Part model, mm, in its own coordinate system. A direction names the side the tool comes from. Coordinates: 2 decimals unless noted, no trailing zeros. Loops run counter-clockwise (first coordinate to the right, second up) from the corner with the lowest first, then second, coordinate; pieces in that order, holes last. Notation, with made-up numbers: (-29.75, 81.5) - (25.25, 81.5) arc R26 ccw to (25.25, 111.5) - close; hole circle Ø9 at (81, 89.25). An arc over 180 degrees is marked (long way). Answer as CSV lines item,"result".
from build123d import *

# Parameters (mm, degrees)
BOSS_EXTRUDE1_DEPTH     = 5
BOSS_EXTRUDE1_DRAFT     = 20
MIRROR1_COPY_1_DEPTH    = 5
MIRROR1_COPY_1_DRAFT    = 20
FILLET1_R               = 10
CUT_EXTRUDE1_DEPTH      = 0.5
SKETCH3_R               = 3.628485538
CUT_EXTRUDE2_DEPTH      = 1
CUT_EXTRUDE2_DRAFT      = -20
SKETCH4_W               = 69.290584113
SKETCH4_H               = 7.5
BOSS_EXTRUDE2_DEPTH     = 25
CUT_EXTRUDE3_DEPTH      = 79.012436871
CUT_EXTRUDE3_DEPTH_BACK = 70


with BuildPart() as part:
    # Sketch1 → Boss-Extrude1 (with draft: the straight prism first)
    with BuildSketch(Plane.XY):
        with BuildLine():
            ThreePointArc((-20.793357934, 20), (-40.793357934, 0), (-20.793357934, -20))
            Line((-20.793357934, -20), (9.206642066, -20))
            ThreePointArc((9.206642066, -20), (29.206642066, 0), (9.206642066, 20))
            Line((9.206642066, 20), (-20.793357934, 20))
        make_face()
    extrude(amount=-BOSS_EXTRUDE1_DEPTH)
    # Boss-Extrude1: the draft: its side faces are tilted about the plane it starts from
    boss_extrude1_sides = [part.faces().sort_by_distance(p)[0] for p in [
        (-5.793357934, -20, -2.5),
        (29.206642066, 0, -2.5),
        (-5.793357934, 20, -2.5),
        (-40.793357934, 0, -2.5),
    ]]
    draft(boss_extrude1_sides, Plane.XY, BOSS_EXTRUDE1_DRAFT)


with BuildPart() as mirror1_copy_1_tool:
    # Mirror1 copy 1 sketch → Mirror1 copy 1 (with draft: the straight prism first)
    with BuildSketch(Plane(origin=(0, 0, -10), x_dir=(1, 0, 0), z_dir=(0, 0, -1))):
        with BuildLine():
            ThreePointArc((-20.793357934, -20), (-40.793357934, 0), (-20.793357934, 20))
            Line((-20.793357934, 20), (9.206642066, 20))
            ThreePointArc((9.206642066, 20), (29.206642066, 0), (9.206642066, -20))
            Line((9.206642066, -20), (-20.793357934, -20))
        make_face()
    extrude(amount=-MIRROR1_COPY_1_DEPTH)
    # Mirror1 copy 1: the draft: its side faces are tilted about the plane it starts from
    mirror1_copy_1_sides = [mirror1_copy_1_tool.faces().sort_by_distance(p)[0] for p in [
        (-5.793357934, -20, -7.5),
        (29.206642066, 0, -7.5),
        (-5.793357934, 20, -7.5),
        (-40.793357934, 0, -7.5),
    ]]
    draft(mirror1_copy_1_sides, Plane(origin=(0, 0, -10), x_dir=(1, 0, 0), z_dir=(0, 0, -1)), MIRROR1_COPY_1_DRAFT)


with BuildPart() as part_1:
    add(part.part)

    # Mirror1 copy 1: add mirror1_copy_1_tool
    add(mirror1_copy_1_tool.part)

    # Fillet1
    fillet1_edges = [part_1.edges().sort_by_distance(p)[0] for p in [
        (31.026493238, 0, -5),
        (-5.793357934, 21.819851171, -5),
        (-42.613209105, 0, -5),
        (-5.793357934, -21.819851171, -5),
    ]]
    fillet(fillet1_edges, radius=FILLET1_R)

    # Sketch2 → Cut-Extrude1 (cut)
    with BuildSketch(Plane(origin=(0, 0, -10), x_dir=(-1, 0, 0), z_dir=(0, 0, -1))):
        with BuildLine():
            Line((-17.429161642, 6.728379016), (-2.895862967, 6.728379016))
            ThreePointArc((-2.895862967, 6.728379016), (3.832516049, 0), (-2.895862967, -6.728379016))
            Line((-2.895862967, -6.728379016), (-17.429161642, -6.728379016))
            ThreePointArc((-17.429161642, -6.728379016), (-24.157540659, 0), (-17.429161642, 6.728379016))
        make_face()
    extrude(amount=-CUT_EXTRUDE1_DEPTH, mode=Mode.SUBTRACT)


with BuildPart() as cut_extrude2_tool:
    # Sketch3 → Cut-Extrude2 (with draft: the straight prism first)
    with BuildSketch(Plane(origin=(0, 0, -9.5), x_dir=(-1, 0, 0), z_dir=(0, 0, -1))):
        with Locations((-17.44999147, 0)):
            Circle(SKETCH3_R)
    extrude(amount=-CUT_EXTRUDE2_DEPTH)
    # Cut-Extrude2: the draft: its side faces are tilted about the plane it starts from
    cut_extrude2_sides = [cut_extrude2_tool.faces().sort_by_distance(p)[0] for p in [
        (21.078477008, 0, -9),
    ]]
    draft(cut_extrude2_sides, Plane(origin=(0, 0, -9.5), x_dir=(-1, 0, 0), z_dir=(0, 0, -1)), CUT_EXTRUDE2_DRAFT)


with BuildPart() as part_2:
    add(part_1.part)

    # Cut-Extrude2: cut by cut_extrude2_tool
    add(cut_extrude2_tool.part, mode=Mode.SUBTRACT)

    # Sketch4 → Boss-Extrude2 (add)
    with BuildSketch(Plane.XY):
        with Locations((-5.793357933, 0)):
            Rectangle(SKETCH4_W, SKETCH4_H)
    extrude(amount=BOSS_EXTRUDE2_DEPTH)

    # Sketch5 → Cut-Extrude3 (cut, two sides: drawn at the far end of the back side and taken through both)
    with BuildSketch(Plane.ZY.offset(40.43864999).offset(-CUT_EXTRUDE3_DEPTH_BACK)):
        with BuildLine():
            Line((118.957682206, 2), (25, 2))
            ThreePointArc((25, 2), (23, 0), (25, -2))
            Line((25, -2), (118.957682206, -2))
            Line((118.957682206, -2), (306.873046617, -2))
            Line((306.873046617, -2), (306.873046617, 2))
            Line((306.873046617, 2), (118.957682206, 2))
        make_face()
    extrude(amount=CUT_EXTRUDE3_DEPTH + CUT_EXTRUDE3_DEPTH_BACK, mode=Mode.SUBTRACT)


solid = part_2.part
Q1. Saw through at A-A (z = 8). Give the cut face in (x, y), then the cut area to 3 significant figures.
Results:
outline,"(-40.44, -3.75) - (28.85, -3.75) - (28.85, 3.75) - (-40.44, 3.75) - close"
area,"520 mm^2"
Q2. Wall check: L1, parallel to Z at x = -2.5, y = -8.5; L2, parallel to Y at x = -15, z = 2; L3, parallel to X at y = 1.5, z = 7. Give the ranges that are in metal, low to high.
Results:
L1,"z = -10 to 0"
L2,"y = -3.75 to 3.75"
L3,"x = -40.44 to 28.85"
Q3. Two-plate mould, pull along Y, no slides. Class faces 5 (the face through (24.156, -0.148, -9.754)), 6 (the face through (-6, 12, 0)), 7 (the face through (-40.9, 0.4, -0.3)): released by +Y, released by -Y, zero draft, split by the parting line, or undercut.
Results:
face 5,"undercut"
face 6,"zero draft"
face 7,"split by the parting line"
Q4. Flat gauge pins, fed straight in: pin 1 (5 mm diameter, centred on x = 19, y = -1, fed in from -Z); pin 2 (8 mm diameter, centred on x = -19.5, y = -10.5, fed in from +Z); pin 3 (1.5 mm diameter, centred on x = -34.5, z = -2, fed in from +Y); pin 4 (12 mm diameter, centred on x = 8.5, z = -3.5, fed in from +Y). Where does each tip first touch, or does it go through?
Results:
pin 1,"stops at z = -9.5"
pin 2,"stops at z = 0"
pin 3,"stops at y = 16.23"
pin 4,"stops at y = 21.18"
Q5. Which spindle directions (+Z, -Z, +X, -X, +Y, -Y) get a long thin tool onto all of the face, cutting with end or side? Do faces 1 (the face through (17, 0, -8.5)), 2 (the face through (-6, 3.75, 12)), 3 (the face through (-6, -12, 0)), 4 (the face through (-40.439, 0, 12)). Say none if no direction does.
Results:
face 1,"-Z"
face 2,"+Z, +X, -X, +Y"
face 3,"+Z, +X, -X, -Y"
face 4,"+Z, -X, +Y, -Y"
